from build123d import *

# Parameters (mm, degrees)
SKETCH1_W           = 75
SKETCH1_H           = 48
BOSS_EXTRUDE1_DEPTH = 48
SHELL1_T            = -1.5
SKETCH2_W           = 30
SKETCH2_H           = 25
CUT_EXTRUDE2_DEPTH  = 50
SKETCH3_W           = 30
SKETCH3_H           = 10
CUT_EXTRUDE3_DEPTH  = 15
SKETCH4_W           = 20
SKETCH4_H           = 25
CUT_EXTRUDE4_DEPTH  = 15
SKETCH5_W           = 7
SKETCH5_H           = 2
CUT_EXTRUDE5_DEPTH  = 15


with BuildPart() as part:
    # Sketch1 → Boss-Extrude1 (new body)
    with BuildSketch(Plane(origin=(0, 0, 0), x_dir=(1, 0, 0), z_dir=(0, 1, 0))):
        with Locations((37.5, 24)):
            Rectangle(SKETCH1_W, SKETCH1_H)
    extrude(amount=BOSS_EXTRUDE1_DEPTH)

    # Shell1
    shell1_openings = [part.faces().sort_by_distance(p)[0] for p in [
        (37.5, 48, -24),
    ]]
    offset(amount=SHELL1_T, openings=shell1_openings, kind=Kind.INTERSECTION)

    # Sketch2 → Cut-Extrude2 (cut)
    with BuildSketch(Plane(origin=(75, 0, 0), x_dir=(0, 0, -1), z_dir=(1, 0, 0))):
        with Locations((31.5, 14)):
            Rectangle(SKETCH2_W, SKETCH2_H)
    extrude(amount=-CUT_EXTRUDE2_DEPTH, mode=Mode.SUBTRACT)

    # Sketch3 → Cut-Extrude3 (cut)
    with BuildSketch(Plane.XZ):
        with Locations((37.5, -5)):
            Rectangle(SKETCH3_W, SKETCH3_H)
    extrude(amount=-CUT_EXTRUDE3_DEPTH, mode=Mode.SUBTRACT)

    # Sketch4 → Cut-Extrude4 (cut)
    with BuildSketch(Plane.ZY):
        with Locations((-11.5, 14)):
            Rectangle(SKETCH4_W, SKETCH4_H)
    extrude(amount=-CUT_EXTRUDE4_DEPTH, mode=Mode.SUBTRACT)

    # Sketch5 → Cut-Extrude5 (cut)
    with BuildSketch(Plane(origin=(0, 0, -48), x_dir=(-1, 0, 0), z_dir=(0, 0, -1))):
        with Locations((-37.5, 19.75)):
            Rectangle(SKETCH5_W, SKETCH5_H)
        with Locations((-37.5, 39.75)):
            Rectangle(SKETCH5_W, SKETCH5_H)
    extrude(amount=-CUT_EXTRUDE5_DEPTH, mode=Mode.SUBTRACT)


solid = part.part
The model under review builds one solid part; all positions refer to its coordinate system, in mm. A direction names the side the tool comes from. Give positions to 0.01 mm unless a question says otherwise; leave off trailing zeros. Write each loop counter-clockwise with the first axis right and the second up, starting at its lowest first coordinate (ties: lowest second). Pieces come first, ordered by that corner, then holes.
1. For P1, Ø1, axis at x = 64.5, y = 34, coming from the +Z side; P2, Ø2, axis at x = 30, z = -22, coming from the +Y side; P3, Ø8, axis at y = 16, z = -25.5, coming from the +X side, all flat-tipped, find the tip position at first contact; note any pin that passes through.
2. Draft analysis for pull direction X (two halves, no side actions). For faces 1 (the flat face through (1.5, 30, -29)), 2 (the flat face through (0, 29, -29)), 3 (the flat face through (37, 1.5, -24)), state which applies: +X half, -X half, draft (parallel to the pull), parting line (faces both ways), or undercut.
3. Add section C-C, the plane x = 24. Write out the cut boundary in (y, z), plus the area to 3 significant figures.
4. Tool access review of faces 4 (the flat face through (52.5, 5, -1)), 5 (the flat face through (73.5, 30, -19)), 6 (the flat face through (75, 29, -18)): name each direction out of +Z, -Z, +X, -X, +Y, -Y from which nothing blocks a thin tool from reaching the whole face with its end or side.
5. Add section D-D, the plane y = 29. Write out the cut boundary in (x, z), plus the area to 3 significant figures.
6. Wall thickness on L1, parallel to Z at x = 24, y = 30; L2, parallel to X at y = 36, z = -30.5; L3, parallel to X at y = 26, z = -23.5: over which ranges is each line inside the solid? List them lowest first.
7. Add section A-A, the plane y = 22. Write out the cut boundary in (x, z), plus the area to 3 significant figures.
8. Add section B-B, the plane z = -8. Write out the cut boundary in (x, y).
Worked answers:
1. P1: stops at z = 0
1. P2: stops at y = 1.5
1. P3: stops at x = 1.5
2. face 1: undercut
2. face 2: -X half
2. face 3: draft
3. outline: (0, -48) - (48, -48) - (48, -46.5) - (1.5, -46.5) - (1.5, -10) - (0, -10) - close; (15, -1.5) - (48, -1.5) - (48, 0) - (15, 0) - close
3. area: 176 mm2
4. face 4: +Z, -Y
4. face 5: +Y
4. face 6: +Z, -Z, +X, +Y, -Y
5. outline: (0, -48) - (75, -48) - (75, 0) - (0, 0) - close; hole (1.5, -46.5) - (73.5, -46.5) - (73.5, -1.5) - (1.5, -1.5) - close
5. area: 360 mm2
6. L1: z = -48 to -46.5, -1.5 to 0
6. L2: x = 0 to 1.5, 73.5 to 75
6. L3: x = 0 to 1.5
7. outline: (0, -48) - (75, -48) - (75, -46.5) - (1.5, -46.5) - (1.5, -21.5) - (0, -21.5) - close; (0, -1.5) - (73.5, -1.5) - (73.5, -16.5) - (75, -16.5) - (75, 0) - (0, 0) - close
7. area: 285 mm2
8. outline: (0, 0) - (22.5, 0) - (22.5, 1.5) - (0, 1.5) - close; (0, 26.5) - (1.5, 26.5) - (1.5, 48) - (0, 48) - close; (52.5, 0) - (75, 0) - (75, 48) - (73.5, 48) - (73.5, 1.5) - (52.5, 1.5) - close
